from build123d import *

# Parameters (mm, degrees)
BOSS_EXTRU_1_DEPTH = 10
BOSS_EXTRU_2_REACH = 312.393
ESQUISSE2_W        = 5
ESQUISSE2_H        = 24
CONG_1_RADIUS      = 12
CONG_1_LENGTH      = 10
BOSS_EXTRU_3_START = -19
ESQUISSE3_W        = 10
ESQUISSE3_H        = 10
ESQUISSE3_R        = 1.5
BOSS_EXTRU_3_DEPTH = 5
CONG_2_R           = 10
CONG_3_R           = 10
CONG_4_R           = 2.5
CONG_5_R           = 2.5
CONG_6_R           = 5


# Some blends are built 0.0001 mm under size
with BuildPart() as part:
    # Esquisse1 → Boss.-Extru.1 (new body)
    with BuildSketch(Plane.XY):
        Polygon((-150, 7), (-155, 7), (-155, -12), (155, -12), (155, -7), (150, -7), (-150, -7), align=None)
        Polygon((155, 12), (-155, 12), (-155, 7), (-150, 7), (150, 7), (155, 7), align=None)
    extrude(amount=BOSS_EXTRU_1_DEPTH)

    # Esquisse2 → Boss.-Extru.2 (add, up to next)
    with BuildSketch(Plane(origin=(155, 0, 0), x_dir=(0, 0, -1), z_dir=(1, 0, 0)), mode=Mode.PRIVATE) as boss_extru_2_sk1:
        with Locations((-7.5, 0)):
            Rectangle(ESQUISSE2_W, ESQUISSE2_H)
    boss_extru_2_tool1 = extrude(boss_extru_2_sk1.sketch, amount=-BOSS_EXTRU_2_REACH, mode=Mode.PRIVATE) - part.part
    add(boss_extru_2_tool1.solids().sort_by_distance((155, 0, 7.5))[0])

    # Congé1: full round fillet: the end face becomes a half cylinder, R = half its width
    cong_1_face = Plane((-155, 0, 5), x_dir=(0, 0, 1), z_dir=(-1, 0, 0))  # on the end face: x along it, z out of the body
    cong_1_slab = cong_1_face.offset(-CONG_1_RADIUS / 2) * Box(CONG_1_LENGTH, 2 * CONG_1_RADIUS, CONG_1_RADIUS, mode=Mode.PRIVATE)  # the body's end, R deep
    cong_1_round = Plane((-143, 0, 5), x_dir=(-1, 0, 0), z_dir=(0, 0, 1)) * Cylinder(CONG_1_RADIUS, CONG_1_LENGTH, mode=Mode.PRIVATE)  # its axis R under the face
    add(cong_1_slab - cong_1_round, mode=Mode.SUBTRACT)

    # Esquisse3 → Boss.-Extru.3 (add)
    # profile 1 of 3: a face of its own
    with BuildSketch(Plane.XZ.offset(12).offset(BOSS_EXTRU_3_START)):
        with Locations((-8, 15)):
            Rectangle(ESQUISSE3_W, ESQUISSE3_H)
        with Locations(Location((-8, 15, 0), (0, 0, 270))):
            Circle(ESQUISSE3_R, mode=Mode.SUBTRACT)
    # profile 2 of 3: a face of its own
    with BuildSketch(Plane.XZ.offset(12).offset(BOSS_EXTRU_3_START)):
        with Locations((-138, 15)):
            Rectangle(ESQUISSE3_W, ESQUISSE3_H)
        with Locations(Location((-138, 15, 0), (0, 0, 270))):
            Circle(ESQUISSE3_R, mode=Mode.SUBTRACT)
    # profile 3 of 3: a face of its own
    with BuildSketch(Plane.XZ.offset(12).offset(BOSS_EXTRU_3_START)):
        with Locations((122, 15)):
            Rectangle(ESQUISSE3_W, ESQUISSE3_H)
        with Locations(Location((122, 15, 0), (0, 0, 270))):
            Circle(ESQUISSE3_R, mode=Mode.SUBTRACT)
    extrude(amount=-BOSS_EXTRU_3_DEPTH)

    # Congé2
    # the kernel refuses this fillet: 10 mm, written as the material it adds along each edge
    with BuildSketch(Plane(origin=(-143, 7, 10), x_dir=(-1, 0, 0), z_dir=(0, 1, 0))) as cong_2_piece_1_section:
        with BuildLine():
            CenterArc((CONG_2_R, CONG_2_R), CONG_2_R, 180, 90)
            Line((0, CONG_2_R), (0, 0))
            Line((0, 0), (CONG_2_R, 0))
        make_face()
    cong_2_piece_1 = extrude(amount=30, mode=Mode.PRIVATE)
    cong_2_piece_1 = cong_2_piece_1 & Plane(origin=(-143, 0, 12.346007959), x_dir=(-1, 0, 0), z_dir=(0, 0, 1)) * Cylinder(12, 100, mode=Mode.PRIVATE)
    add(cong_2_piece_1)

    # Congé3
    cong_3_edges = [part.edges().sort_by_distance(p)[0] for p in [
        (127, 9.5, 10),
        (117, 9.5, 10),
        (-3, 9.5, 10),
        (-13, 9.5, 10),
        (-133, 9.5, 10),
    ]]
    fillet(cong_3_edges, radius=CONG_3_R - 0.0001)  # a hair under: the kernel refuses the full size

    # Congé4
    cong_4_edges = [part.edges().sort_by_distance(p)[0] for p in [
        (155, -12, 5),
        (155, -7, 2.5),
    ]]
    fillet(cong_4_edges, radius=CONG_4_R - 0.0001)  # a hair under: the kernel refuses the full size

    # Congé5
    cong_5_edges = [part.edges().sort_by_distance(p)[0] for p in [
        (155, 12, 5),
        (155, 7, 2.5),
    ]]
    fillet(cong_5_edges, radius=CONG_5_R - 0.0001)  # a hair under: the kernel refuses the full size

    # Congé6
    cong_6_edges = [part.edges().sort_by_distance(p)[0] for p in [
        (-143, 9.5, 20),
        (-133, 9.5, 20),
        (-13, 9.5, 20),
        (-3, 9.5, 20),
        (117, 9.5, 20),
        (127, 9.5, 20),
    ]]
    fillet(cong_6_edges, radius=CONG_6_R)


solid = part.part
The model under review builds one solid part; all positions refer to its coordinate system, in mm. A direction names the side the tool comes from. Give positions to 0.01 mm unless a question says otherwise; leave off trailing zeros. Order: outer loops, then holes, each group sorted by start corner. A loop starts at its lowest first (then second) coordinate and runs counter-clockwise, first axis right, second up. Notation, with made-up numbers: (66, 45) -> (75, 45) arc R19 cw to (75, 49) -> close; hole circle Ø7 at (18, 67). An arc over 180 degrees is marked (long way). Write item = value, one per line. Start each with the question number.
(1) Take a section at B-B (y = 0). Write out the cut boundary in (x, z), plus the area to 4 significant figures.
(2) Draft analysis for pull direction Y (two halves, no side actions). For faces 6 (the cylindrical face through (1, 10, 12)), 7 (the cylindrical face through (-155, 0, 5)), 8 (the flat face through (-150, 0, 2)), state which applies: +Y half, -Y half, draft (parallel to the pull), parting line (faces both ways), or undercut.
(3) For L1, parallel to Z at x = 122, y = 9.35; L2, parallel to X at y = 9.05, z = 15; L3, parallel to X at y = 9.75, z = 18.5, list the stretches that pass through material, from the lowest coordinate up. Write a range as from..to.
(4) Tool access review of faces 1 (the cylindrical face through (-17, 10, 12)), 2 (the flat face through (2, 0, 10)), 3 (the cylindrical face through (131, 10, 12)), 4 (the flat face through (3, -7, 2)), 5 (the flat face through (122, 7, 13)): name each direction out of +Z, -Z, +X, -X, +Y, -Y from which nothing blocks a thin tool from reaching the whole face with its end or side.
(5) For pin 1 Ø8 at (x, y) = (81, -7.5) entering from +Z; pin 2 Ø5 at (y, z) = (3, 15) entering from +X; pin 3 Ø1.5 at (y, z) = (-7, 7) entering from -X; pin 4 Ø5.5 at (y, z) = (0, 1.5) entering from +X, all flat-tipped, find the tip position at first contact; note any pin that passes through.
(6) Take a section at A-A (x = -64). Write out the cut boundary in (y, z), plus the area to 3 significant figures.
Returned:
q1.outline = (-155, 0) -> (-150, 0) -> (-150, 5) -> (155, 5) -> (155, 10) -> (-155, 10) -> close
q1.area = 1,575 mm²
q2.face_6 = draft
q2.face_7 = parting line
q2.face_8 = undercut
q3.L1 = 0..13.5, 16.5..20
q3.L2 = -144.34..-139.5, -136.5..-131.66, -14.34..-9.5, -6.5..-1.66, 115.66..120.5, 123.5..128.34
q3.L3 = -142.43..-133.57, -12.43..-3.57, 117.57..126.43
q4.face_1 = +Z, +Y, -Y
q4.face_2 = +Z, -Y
q4.face_3 = +Z, +X, +Y, -Y
q4.face_4 = -Z, +X
q4.face_5 = +Z, +X, -X, -Y
q5.pin_1 = 10
q5.pin_2 = through
q5.pin_3 = -153.24
q5.pin_4 = -150
q6.outline = (-12, 0) -> (-7, 0) -> (-7, 5) -> (7, 5) -> (7, 0) -> (12, 0) -> (12, 10) -> (-12, 10) -> close
q6.area = 170 mm²
